Build history of the part. All positions in model axes, mm. Face numbers are marked on the shaded views. Coordinates: 2 decimals unless noted, no trailing zeros. Order: outer loops, then holes, each group sorted by start corner. A loop starts at its lowest first (then second) coordinate and runs counter-clockwise, first axis right, second up. Notation, with made-up numbers: (35, 35) - (85, 35) arc R19 cw to (85, 71) - close; hole circle Ø9 at (34.25, 52). An arc over 180 degrees is marked (long way). Return JSON: item names as keys, results as strings.
from build123d import *

# Parameters (mm, degrees)
SKETCH007_W            = 250
SKETCH007_H            = 65
PAD004_DEPTH           = 3
SKETCH015_R            = 1.4
POCKET007_DEPTH        = 5
SKETCH032_W            = 10
SKETCH032_H            = 8
PAD011_DEPTH           = 6
SKETCH033_R            = 1.228205
SKETCH033_R_2          = 1.080341
POCKET017_DEPTH        = 65.001
SKETCH036_R            = 5
SKETCH036_R_2          = 1.4
SKETCH036_R_3          = 5.456257
SKETCH036_W            = 210
SKETCH036_H            = 4
PAD013_DEPTH           = 2
SKETCH037_W            = 15
SKETCH037_H            = 3
POCKET019_DEPTH        = 5
LINEARPATTERN002_COUNT = 6
LINEARPATTERN002_PITCH = 36.8
SKETCH044_W            = 2
SKETCH044_H            = 2
PAD017_DEPTH           = 250
CHAMFER025_SIZE        = 1.5


with BuildPart() as part:
    # Sketch007 → Pad004 (new body)
    with BuildSketch(Plane.XZ):
        Rectangle(SKETCH007_W, SKETCH007_H)
    extrude(amount=PAD004_DEPTH)

    # Sketch015 (on Face5 of Pad004) → Pocket007 (cut)
    with BuildSketch(Plane(origin=(0, 0, 0), x_dir=(1, 0, 0), z_dir=(0, 1, 0))):
        with Locations((-113.5, 15)):
            Circle(SKETCH015_R)
        with Locations((113.5, -15)):
            Circle(SKETCH015_R)
    extrude(amount=-POCKET007_DEPTH, mode=Mode.SUBTRACT)

    # Sketch032 (on Face1 of Pocket007) → Pad011 (join)
    with BuildSketch(Plane(origin=(0, 0, 32.5), x_dir=(-1, 0, 0), z_dir=(0, 0, 1))):
        with Locations((-50, 5)):
            Rectangle(SKETCH032_W, SKETCH032_H)
        with Locations((50, 5)):
            Rectangle(SKETCH032_W, SKETCH032_H)
    pad011 = extrude(amount=-PAD011_DEPTH)

    # Mirrored: Pad011 across XY
    add(pad011.mirror(Plane.XY))

    # Sketch033 (on Face23 of Mirrored) → Pocket017 (cut, through all)
    with BuildSketch(Plane(origin=(0, 0, 32.5), x_dir=(-1, 0, 0), z_dir=(0, 0, 1))):
        with Locations((-50, 5)):
            Circle(SKETCH033_R)
        with Locations((50, 5)):
            Circle(SKETCH033_R_2)
    extrude(amount=-POCKET017_DEPTH, mode=Mode.SUBTRACT)

    # Sketch036 (on Face4 of Pocket017) → Pad013 (join)
    with BuildSketch(Plane.XZ.offset(3)):
        with Locations((-113.49704, -14.99673)):
            Circle(SKETCH036_R)
        with Locations((-113.49704, -14.99673)):
            Circle(SKETCH036_R_2, mode=Mode.SUBTRACT)
        with Locations((113.510239, 14.966872)):
            Circle(SKETCH036_R)
        with Locations((113.510239, 14.966872)):
            Circle(SKETCH036_R_2, mode=Mode.SUBTRACT)
        Circle(SKETCH036_R_3)
        with Locations((-0.3682397708, 14)):
            Rectangle(SKETCH036_W, SKETCH036_H)
        with Locations((0.3682397708, -14)):
            Rectangle(SKETCH036_W, SKETCH036_H)
    extrude(amount=PAD013_DEPTH)

    # Sketch037 (on Face4 of Pad013) → Pocket019 (cut)
    with BuildSketch(Plane.XZ.offset(3)):
        with Locations((-92.5, -0.19377)):
            Rectangle(SKETCH037_W, SKETCH037_H)
    pocket019 = extrude(amount=-POCKET019_DEPTH, mode=Mode.SUBTRACT)

    # LinearPattern002: Pocket019 ×6
    with Locations(*[(i * LINEARPATTERN002_PITCH, 0, 0) for i in range(1, LINEARPATTERN002_COUNT)]):
        add(pocket019, mode=Mode.SUBTRACT)

    # Sketch044 (on Face7 of MultiTransform001) → Pad017 (join)
    with BuildSketch(Plane(origin=(-125, 0, 0), x_dir=(0, 0, -1), z_dir=(-1, 0, 0))):
        with Locations((-33.5, 1)):
            Rectangle(SKETCH044_W, SKETCH044_H)
    pad017 = extrude(amount=-PAD017_DEPTH)

    # Mirrored003: Pad017 across Sketch044 V_Axis
    add(pad017.mirror(Plane(origin=(-125, 0, 0), x_dir=(-1, 0, 0), z_dir=(0, 0, -1))))

    # Chamfer025
    chamfer025_edges = [part.edges().sort_by_distance(p)[0] for p in [
        (125, -1, -34.5),
        (125, -1, 34.5),
        (-125, -1, 34.5),
        (-125, -1, -34.5),
    ]]
    chamfer(chamfer025_edges, length=CHAMFER025_SIZE)


with BuildPart() as part_1:
    # Body003 placement: moved
    add(part.part.moved(Location((0, 80, 0))))


solid = part_1.part
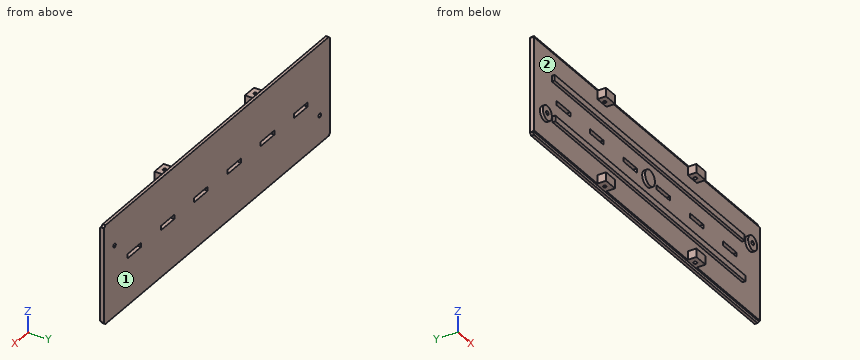
1. Probe L1, parallel to X at y = 74.75, z = 30.5; L2, parallel to Y at x = 50, z = 28.15; L3, parallel to Z at x = 60.5, y = 78.75. List the from-to ranges inside material, lowest first.
Check values:
{"L1": "-55 to -51.05, -48.95 to -45, 45 to 48.8, 51.2 to 55", "L2": "71 to 73.77, 76.23 to 80", "L3": "-34.5 to -1.69, 1.31 to 34.5"}
2. Drop flat-ended pins along their axis: pin 1 (1.6 mm diameter, centred on y = 75.5, z = 13, fed in from +X); pin 2 (4 mm diameter, centred on x = -83.5, y = 77, fed in from +Z); pin 3 (1.8 mm diameter, centred on x = -49.5, y = 74.5, fed in from +Z); pin 4 (1.7 mm diameter, centred on x = -50, y = 75, fed in from +Z). Give the stop position or say it passes through.
Check values:
{"pin 1": "x = 118.37", "pin 2": "z = 34.5", "pin 3": "z = 32.5", "pin 4": "z = 16"}
3. Cut at B-B on x = -69.5. Give the cut face in (y, z), plus the area to 3 significant figures.
Check values:
{"outline": "(75, -16) - (77, -16) - (77, -32.5) - (78, -32.5) - (78, -34.5) - (80, -34.5) - (80, 34.5) - (78, 34.5) - (78, 32.5) - (77, 32.5) - (77, 16) - (75, 16) - (75, 12) - (77, 12) - (77, -12) - (75, -12) - close", "area": "219 mm²"}
4. Mould opens along Z. For the marked faces 1 and 2 say: pulls with the +Z half, pulls with the -Z half, needs draft (parallel to the pull), parting line crosses it, or undercut.
Check values:
{"face 1": "needs draft", "face 2": "undercut"}
5. Cut at A-A on x = -19. Give the cut face in (y, z).
Check values:
{"outline": "(75, -16) - (77, -16) - (77, -32.5) - (78, -32.5) - (78, -34.5) - (80, -34.5) - (80, -1.69) - (77, -1.69) - (77, -12) - (75, -12) - close; (75, 12) - (77, 12) - (77, 1.31) - (80, 1.31) - (80, 34.5) - (78, 34.5) - (78, 32.5) - (77, 32.5) - (77, 16) - (75, 16) - close"}
